CAD build for the part. Positions are in the model's coordinates, mm. A direction names the side the tool comes from. Coordinates: 2 decimals unless noted, no trailing zeros. Order: outer loops, then holes, each group sorted by start corner. A loop starts at its lowest first (then second) coordinate and runs counter-clockwise, first axis right, second up. Notation, with made-up numbers: M 73.25,41 L 124.25,41 A19 cw 124.25,74 Z; hole C 32.25,68 d2. An arc over 180 degrees is marked long. One line per item, written item: value.
Autodesk Inventor part; units mm, degrees
ref_plane "YZ Plane" through (0, 0, 0) normal (1, 0, 0) x (0, 1, 0)
ref_plane "XY Plane" through (0, 0, 0) normal (0, 0, 1) x (1, 0, 0)
sketch "Sketch1" plane through (0, 0, 0) normal (0, 1, 0) x (-1, 0, 0)
  arc A0 (0, -11) -> (0, 11) centre (0, 0) ccw
  line L0 (0, 0) -> (0, -11) construction
  line L1 (0, 0) -> (0, 11) construction
  arc A1 (0, -14) -> (0, 14) centre (0, 0) ccw
  line L2 (0, 11) -> (0, 14)
  line L3 (0, -11) -> (0, -14)
  dimension "d0" = 180
  dimension "d1" = 11
  dimension "d3" = 3
extrude "Extrusion1" add sketch "Sketch1" along normal mid plane 20
sketch "Sketch2" plane through (0, 10, 0) normal (0, 1, 0) x (1, 0, 0)
  arc A0 (0, 14) -> (0, -14) centre (0, 0) ccw
  arc A1 (0, 11) -> (0, -11) centre (0, 0) ccw construction
  arc A2 (0, 7) -> (0, -7) centre (0, 0) ccw
  line L0 (0, 11) -> (0, 14)
  line L1 (0, 14) -> (0, 7)
  line L2 (0, -7) -> (0, -14)
  dimension "d6" = 4
extrude "Extrusion2" add sketch "Sketch2" along normal blind 4
sketch "Sketch3" plane through (0, -10, 0) normal (0, -1, 0) x (1, 0, 0)
  arc A0 (0, 14) -> (0, -14) centre (0, 0) ccw
  line L0 (0, 14) -> (0, 7)
  arc A1 (0, 7) -> (0, -7) centre (0, 0) ccw
  line L1 (0, -7) -> (0, -14)
  arc A2 (0, 14) -> (0, -14) centre (0, 0) ccw
  point P0 (0, -14)
extrude "Extrusion3" add sketch "Sketch3" along normal blind 4
ref_plane "Work Plane1" through (0, 4, 0) normal (0, 1, 0) x (-1, 0, 0)
sketch "Sketch4" plane through (0, 4, 0) normal (0, 1, 0) x (-1, 0, 0)
  arc A0 (0, -14) -> (0, 14) centre (0, 0) ccw
  arc A1 (0, -20.5) -> (0, 20.5) centre (0, 0) ccw
  line L0 (0, 20.5) -> (0, 14)
  line L1 (0, -14) -> (0, -20.5)
  circle A2 centre (17.25, 0) radius 1.5
  line L2 (14, 0) -> (20.5, 0) construction
  circle A3 centre (8.625, 14.9389) radius 1.5
  circle A4 centre (8.625, -14.9389) radius 1.5
  dimension "d12" = 6.5
  dimension "d13" = 3
  dimension "d16" = 60
  dimension "d20" = 60
extrude "Extrusion4" add sketch "Sketch4" along normal blind 4
properties part number "Spindle_Block_Holder" material "PC/ABS Plastic"
Q1. Drill centre lines: line 1 along Y through (x, z) = (-2, -7.5); line 2 along Z through (x, y) = (-8, 5); line 3 along Y through (x, z) = (-5.5, 16). Where is each one in solid material? Low to high.
Recorded:
line 1: y = -14 to -10, 10 to 14
line 2: z = -18.87 to -16.3, -13.58 to -7.55, 7.55 to 13.58, 16.3 to 18.87
line 3: y = 4 to 8
Q2. Pin check, flat tips, straight feed: pin 1 Ø1.5 at (y, z) = (-6.5, -5) entering from +X; pin 2 Ø2 at (y, z) = (10.5, 2.5) entering from -X; pin 3 Ø4 at (y, z) = (4, 16) entering from -X (3 decimals); pin 4 Ø2.5 at (x, z) = (-8.62, -14.94) entering from -Y. Stop position of each tip, or through.
Recorded:
pin 1: stops at x = -9.38
pin 2: stops at x = -13.92
pin 3: stops at x = -14.975
pin 4: passes through
Q3. Mould opens along Z. For faces 4 (the face through (0, 1, -13)), 5 (the face through (-8.43, 5.97, 13.45)), 6 (the face through (-14, 11, 0)) say: released by +Z, released by -Z, zero draft, split by the parting line, or undercut.
Recorded:
face 4: zero draft
face 5: undercut
face 6: split by the parting line
Q4. Slice it at B-B (y = 6.25). List the corners of the cut face in (x, z) (3 decimals), plus the area to 3 significant figures.
Recorded:
outline: M 0,-20.5 L 0,-11 A11 cw 0,11 L 0,20.5 A20.5 ccw Z; hole C -17.25,0 d3; hole C -8.625,-14.939 d3; hole C -8.625,14.939 d3
area: 449 mm^2
Q5. Slice it at C-C (x = -17.25). List the corners of the cut face in (y, z), plus the area to 3 significant figures.
Recorded:
outline: M 4,-11.08 L 8,-11.08 L 8,-1.5 L 4,-1.5 Z; M 4,1.5 L 8,1.5 L 8,11.08 L 4,11.08 Z
area: 76.6 mm^2
Q6. Slice it at A-A (z = 0). List the corners of the cut face in (x, y).
Recorded:
outline: M -20.5,4 L -18.75,4 L -18.75,8 L -20.5,8 Z; M -15.75,4 L -14,4 L -14,-14 L -7,-14 L -7,-10 L -11,-10 L -11,10 L -7,10 L -7,14 L -14,14 L -14,8 L -15.75,8 Z
Q7. Which spindle directions (+Z, -Z, +X, -X, +Y, -Y) get a long thin tool onto all of the face, cutting with end or side? Do faces 1 (the face through (-15, 8, 0)), 2 (the face through (-8, 10, 0)), 3 (the face through (-15, 4, 0)). Say none if no direction does.
Recorded:
face 1: -X, +Y
face 2: +X
face 3: -X, -Y
Q8. Slice it at D-D (z = 15.5). List the corners of the cut face in (x, y), plus the area to 3 significant figures.
Recorded:
outline: M -13.42,4 L -10.02,4 L -10.02,8 L -13.42,8 Z; M -7.23,4 L 0,4 L 0,8 L -7.23,8 Z
area: 42.5 mm^2
